```python
from build123d import *

# Parameters (mm, degrees)
SKETCH1_R           = 1.905
SKETCH1_R_2         = 6.35
BOSS_EXTRUDE1_DEPTH = 6.35
FILLET1_R           = 10


with BuildPart() as part:
    # Sketch1 → Boss-Extrude1 (new body)
    with BuildSketch(Plane.XY):
        Polygon((18.65, -15), (25, -15), (25, -34.5), (27.4, -34.5), (27.4, -33.25), (29.8, -33.25), (29.8, -34.5), (30.65, -34.5), (30.65, -37.5), (29.8, -37.5), (29.8, -38.75), (27.4, -38.75), (27.4, -37.5), (25, -37.5), (25, -59.5), (27.4, -59.5), (27.4, -58.25), (29.8, -58.25), (29.8, -59.5), (30.65, -59.5), (30.65, -62.5), (29.8, -62.5), (29.8, -63.75), (27.4, -63.75), (27.4, -62.5), (25, -62.5), (25, -75), (40, -75), (40, 25), (-25, 25), (-25, -25), (18.65, -25), align=None)
        with Locations((-15.494, -15.494)):
            Circle(SKETCH1_R, mode=Mode.SUBTRACT)
        with BuildLine():
            ThreePointArc((-10.237491978, -12.033543202), (-12.033543202, -12.033543202), (-12.033543202, -10.237491978))
            Line((-12.033543202, -10.237491978), (-9.519071488, -7.723020264))
            ThreePointArc((-9.519071488, -7.723020264), (-7.723020264, -7.723020264), (-7.723020264, -9.519071488))
            Line((-7.723020264, -9.519071488), (-10.237491978, -12.033543202))
        make_face(mode=Mode.SUBTRACT)
        Circle(SKETCH1_R_2, mode=Mode.SUBTRACT)
        with BuildLine():
            ThreePointArc((-12.033543202, 10.237491978), (-12.033543202, 12.033543202), (-10.237491978, 12.033543202))
            Line((-10.237491978, 12.033543202), (-7.723020264, 9.519071488))
            ThreePointArc((-7.723020264, 9.519071488), (-7.723020264, 7.723020264), (-9.519071488, 7.723020264))
            Line((-9.519071488, 7.723020264), (-12.033543202, 10.237491978))
        make_face(mode=Mode.SUBTRACT)
        with Locations((-15.494, 15.494)):
            Circle(SKETCH1_R, mode=Mode.SUBTRACT)
        with Locations((15.494, -15.494)):
            Circle(SKETCH1_R, mode=Mode.SUBTRACT)
        with BuildLine():
            ThreePointArc((12.033543202, -10.237491978), (12.033543202, -12.033543202), (10.237491978, -12.033543202))
            Line((10.237491978, -12.033543202), (7.723020264, -9.519071488))
            ThreePointArc((7.723020264, -9.519071488), (7.723020264, -7.723020264), (9.519071488, -7.723020264))
            Line((9.519071488, -7.723020264), (12.033543202, -10.237491978))
        make_face(mode=Mode.SUBTRACT)
        with BuildLine():
            ThreePointArc((10.237491978, 12.033543202), (12.033543202, 12.033543202), (12.033543202, 10.237491978))
            Line((12.033543202, 10.237491978), (9.519071488, 7.723020264))
            ThreePointArc((9.519071488, 7.723020264), (7.723020264, 7.723020264), (7.723020264, 9.519071488))
            Line((7.723020264, 9.519071488), (10.237491978, 12.033543202))
        make_face(mode=Mode.SUBTRACT)
        with Locations((15.494, 15.494)):
            Circle(SKETCH1_R, mode=Mode.SUBTRACT)
    extrude(amount=BOSS_EXTRUDE1_DEPTH)

    # Fillet1
    fillet1_edges = [part.edges().sort_by_distance(p)[0] for p in [
        (-25, -25, 3.175),
        (-25, 25, 3.175),
        (40, 25, 3.175),
        (40, -75, 3.175),
    ]]
    fillet(fillet1_edges, radius=FILLET1_R)


solid = part.part
```
Geometry check sheet. Reference: the model listing, model coordinates, mm. A direction names the side the tool comes from. Give positions to 0.01 mm unless a question says otherwise; leave off trailing zeros. Loops run counter-clockwise (first coordinate to the right, second up) from the corner with the lowest first, then second, coordinate; pieces in that order, holes last. Notation, with made-up numbers: M 16.5,0 L 32.5,0 A19 ccw 32.5,28 Z; hole C -40,54 d2. An arc over 180 degrees is marked long. Write item = value, one per line. Start each with the question number.
1. Go/stop test with flat-tipped pins: P1, Ø1.5, axis at x = -9.5, z = 2.5, coming from the -Y side; P2, Ø0.9, axis at y = -36, z = 4, coming from the -X side. Record where each tip stops, or that it passes through.
2. Section check D-D, the plane x = 21. Enter the section's corners in (y, z), plus the area to 3 significant figures.
3. Draft check along Y on faces 1 (the face through (25, -48, 3)), 2 (the face through (2, -25, 3)), 3 (the face through (-13.68, 16.07, 3.13)). Enter one of: +Y half, -Y half, draft (parallel to the pull), parting line (faces both ways), or undercut.
4. Thickness scan on probe 1 along Y at (x, z) = (0, 4.5); probe 2 along Y at (x, z) = (-10.5, 4); probe 3 along Y at (x, z) = (8, 1.5). Record the ranges inside material, lowest first.
5. Tool access check on faces 4 (the face through (26, -37.5, 3)), 5 (the face through (-21.99, -22.15, 3.22)), 6 (the face through (18.65, -20, 3)), 7 (the face through (29, -63.75, 3)), 8 (the face through (37.15, -71.99, 3.22)). Record the directions out of +Z, -Z, +X, -X, +Y, -Y that give a thin tool (end or side, any length) a straight path to the whole face; none if there is none.
6. Section check B-B, the plane x = 0. Enter the section's corners in (y, z), plus the area to 3 significant figures.
7. Section check C-C, the plane y = -56. Enter the section's corners in (x, z), plus the area to 4 significant figures.
8. Section check A-A, the plane y = 0. Enter the section's corners in (x, z).
Values follow:
q1.P1 = -25
q1.P2 = 30.65
q2.outline = M -15,0 L 25,0 L 25,6.35 L -15,6.35 Z
q2.area = 254 mm^2
q3.face_1 = draft
q3.face_2 = -Y half
q3.face_3 = undercut
q4.probe_1 = -25 to -6.35, 6.35 to 25
q4.probe_2 = -25 to -12.24, -8.7 to 8.7, 12.24 to 25
q4.probe_3 = -25 to -9.8, -7.51 to 7.51, 9.8 to 25
q5.face_4 = +Z, -Z, -X
q5.face_5 = +Z, -Z, -X, -Y
q5.face_6 = +Z, -Z, -Y
q5.face_7 = +Z, -Z
q5.face_8 = +Z, -Z, +X, -Y
q6.outline = M -25,0 L -6.35,0 L -6.35,6.35 L -25,6.35 Z; M 6.35,0 L 25,0 L 25,6.35 L 6.35,6.35 Z
q6.area = 237 mm^2
q7.outline = M 25,0 L 40,0 L 40,6.35 L 25,6.35 Z
q7.area = 95.25 mm^2
q8.outline = M -25,0 L -6.35,0 L -6.35,6.35 L -25,6.35 Z; M 6.35,0 L 40,0 L 40,6.35 L 6.35,6.35 Z
